Verification items for the finished model (mm, model axes). A direction names the side the tool comes from. Round coordinates to 2 decimals unless told otherwise and drop trailing zeros. Write each loop counter-clockwise with the first axis right and the second up, starting at its lowest first coordinate (ties: lowest second). Pieces come first, ordered by that corner, then holes. Notation, with made-up numbers: (59.25, 10) - (79.25, 10) arc R9 cw to (79.25, 20) - close; hole circle Ø1 at (6, 33.5). An arc over 180 degrees is marked (long way). Answer as a JSON object with one key per item and string values.
```python
from build123d import *

# Parameters (mm, degrees)
F0_W     = 25.4
F0_H     = 25.4
F1_DEPTH = 1.524
F3_DEPTH = 15.24
F2_W     = 5.08
F2_H     = 3.175
F4_DEPTH = 7.62
F9_DEPTH = 12.446
F10_R    = 1.5875


with BuildPart() as f1:
    # F0 (on Top) → F1 (new body)
    with BuildSketch(Plane.XY):
        Rectangle(F0_W, F0_H)
    extrude(amount=F1_DEPTH)

    # F2 (on face) → F3 (join)
    with BuildSketch(Plane.XY.offset(1.524)):
        Polygon((6.223, -6.223), (6.223, 6.223), (3.683, 6.223), (3.683, 1.27), (-3.683, 1.27), (-3.683, 6.223), (-6.223, 6.223), (-6.223, -6.223), (-3.683, -6.223), (-3.683, -1.27), (3.683, -1.27), (3.683, -6.223), align=None)
    extrude(amount=F3_DEPTH)

    # F2 (on face) → F4 (join)
    with BuildSketch(Plane.XY.offset(1.524)):
        with Locations((0, -4.6355)):
            Rectangle(F2_W, F2_H)
        with Locations((0, 4.6355)):
            Rectangle(F2_W, F2_H)
    extrude(amount=F4_DEPTH)

    # F5 (on face) → F6 (revolve)
    with BuildSketch(Plane.XY.offset(9.144)):
        with BuildLine():
            Line((-2.54, 5.08), (2.54, 5.08))
            ThreePointArc((2.54, 5.08), (0, 7.62), (-2.54, 5.08))
        make_face()
    revolve(axis=Axis((0, 5.08, 9.144), (-1, 0, 0)))

    # F5 (on face) → F7 (revolve)
    with BuildSketch(Plane.XY.offset(9.144)):
        with BuildLine():
            ThreePointArc((-2.2682925296, -6.223), (0, -7.62), (2.2682925296, -6.223))
            Line((2.2682925296, -6.223), (-2.2682925296, -6.223))
        make_face()
        with BuildLine():
            ThreePointArc((2.2682925296, -6.223), (2.4711397194, -5.6674253036), (2.54, -5.08))
            Line((2.54, -5.08), (-2.54, -5.08))
            ThreePointArc((-2.54, -5.08), (-2.4711397194, -5.6674253036), (-2.2682925296, -6.223))
            Line((-2.2682925296, -6.223), (2.2682925296, -6.223))
        make_face()
    revolve(axis=Axis((0, -5.08, 9.144), (-1, 0, 0)))

    # F8 (on face) → F9 (join)
    with BuildSketch(Plane(origin=(0, 6.223, 0), x_dir=(-1, 0, 0), z_dir=(0, 1, 0))):
        Polygon((-3.683, 16.764), (-3.683, 10.414), (0, 14.097), (3.683, 10.414), (3.683, 16.764), align=None)
    extrude(amount=-F9_DEPTH)

    # F10
    f10_edges = [f1.edges().sort_by_distance(p)[0] for p in [
        (-6.223, -6.223, 9.144),
        (-6.223, 6.223, 9.144),
        (6.223, 6.223, 9.144),
        (6.223, -6.223, 9.144),
    ]]
    fillet(f10_edges, radius=F10_R)


solid = f1.part
```
1. Go/stop test with flat-tipped pins: pin 1 (7.5 mm diameter, centred on y = 2, z = 7, fed in from +X); pin 2 (4 mm diameter, centred on y = 3, z = 8, fed in from -X); pin 3 (1.5 mm diameter, centred on y = 6, z = 6, fed in from -X). Record where each tip stops, or that it passes through.
Completed:
{"pin 1": "stops at x = 6.22", "pin 2": "stops at x = -6.22", "pin 3": "stops at x = -6.1"}
2. Cross-section at A-A (z = 4.75). Record the boundary of the cut face in (x, y) (1 decimal).
Completed:
{"outline": "(-6.2, -4.6) arc R1.6 ccw to (-4.6, -6.2) - (-3.7, -6.2) - (-3.7, -1.3) - (3.7, -1.3) - (3.7, -6.2) - (4.6, -6.2) arc R1.6 ccw to (6.2, -4.6) - (6.2, 4.6) arc R1.6 ccw to (4.6, 6.2) - (3.7, 6.2) - (3.7, 1.3) - (-3.7, 1.3) - (-3.7, 6.2) - (-4.6, 6.2) arc R1.6 ccw to (-6.2, 4.6) - close; (-2.5, -6.2) - (2.5, -6.2) - (2.5, -3) - (-2.5, -3) - close; (-2.5, 3) - (2.5, 3) - (2.5, 6.2) - (-2.5, 6.2) - close"}
3. Mould release check, pull along Y, two halves, no side actions. Record for faces 1 (the face through (0, -1.27, 6)), 2 (the face through (-2.1, -6.223, 12.4)), 3 (the face through (-6.223, 0, 9)): released by +Y, released by -Y, zero draft, split by the parting line, or undercut.
Completed:
{"face 1": "undercut", "face 2": "released by -Y", "face 3": "zero draft"}
4. Access from +Z, -Z, +X, -X, +Y, -Y to the whole of each face (thin tool, end or side, straight path). Record for faces 4 (the face through (2.54, -5, 5)), 5 (the face through (1.867, 3.781, 12.23)), 6 (the face through (-0.2, -2.6, 1.524)), 7 (the face through (5.77, 5.746, 9.251)).
Completed:
{"face 4": "-Y", "face 5": "+Y", "face 6": "none", "face 7": "+Z, +X, +Y"}
5. Cross-section at C-C (y = 4). Record the boundary of the cut face in (x, z), plus the area to 3 significant figures.
Completed:
{"outline": "(-12.7, 0) - (12.7, 0) - (12.7, 1.52) - (6.22, 1.52) - (6.22, 16.76) - (-6.22, 16.76) - (-6.22, 1.52) - (-12.7, 1.52) - close; hole (-3.68, 1.52) - (-2.54, 1.52) - (-2.54, 9.14) - (-2.3, 9.14) arc R2.3 cw to (2.3, 9.14) - (2.54, 9.14) - (2.54, 1.52) - (3.68, 1.52) - (3.68, 10.41) - (0, 14.1) - (-3.68, 10.41) - close", "area": "196 mm^2"}
6. Cross-section at D-D (y = 0.75). Record the boundary of the cut face in (x, z).
Completed:
{"outline": "(-12.7, 0) - (12.7, 0) - (12.7, 1.52) - (6.22, 1.52) - (6.22, 16.76) - (-6.22, 16.76) - (-6.22, 1.52) - (-12.7, 1.52) - close"}
7. Cross-section at B-B (z = 15.25). Record the boundary of the cut face in (x, y) (1 decimal).
Completed:
{"outline": "(-6.2, -4.6) arc R1.6 ccw to (-4.6, -6.2) - (4.6, -6.2) arc R1.6 ccw to (6.2, -4.6) - (6.2, 4.6) arc R1.6 ccw to (4.6, 6.2) - (-4.6, 6.2) arc R1.6 ccw to (-6.2, 4.6) - close"}
8. Material ranges on probe 1 along X at (y, z) = (3.25, 3.75); probe 2 along X at (y, z) = (6, 8.5); probe 3 along Y at (x, z) = (0, 14.5), recorded low to high. Write a range as from..to.
Completed:
{"probe 1": "x = -6.22..-3.68, -2.54..2.54, 3.68..6.22", "probe 2": "x = -5.45..-3.68, -2.54..2.54, 3.68..5.45", "probe 3": "y = -6.22..6.22"}
